Autodesk Inventor part; units mm, degrees
ref_plane "YZ Plane" through (0, 0, 0) normal (1, 0, 0) x (0, 1, 0)
ref_plane "XZ Plane" through (0, 0, 0) normal (0, 1, 0) x (-1, 0, 0)
ref_plane "XY Plane" through (0, 0, 0) normal (0, 0, 1) x (1, 0, 0)
sketch "Sketch1" plane through (0, 0, 0) normal (0, 1, 0) x (-1, 0, 0)
  line L0 (606, 0) -> (606, -30)
  arc A0 (571.724, -77.4632) -> (606, -30) centre (556, -30) ccw
  arc A1 (0, -169.7009) -> (571.724, -77.4632) centre (0, 1648.2991) ccw
  line L1 (0, 191.6842) -> (0, -191.6842)
  arc A2 (0, -163.7009) -> (569.8371, -71.7676) centre (0, 1648.2991) ccw
  arc A3 (569.8371, -71.7676) -> (600, -30) centre (556, -30) ccw
  line L2 (600, -30) -> (600, 0)
  line L3 (600, 0) -> (606, 0)
  line L4 (0, -163.7009) -> (0, -169.7009)
  point P0 (0, 0)
  point P1 (0, 0)
  point P2 (0, -166.7009)
  point P3 (0, -163.7009)
  point P4 (0, -169.7009)
  dimension "d0" = 50
  dimension "d1" = 30
  dimension "d3" = 1818
  dimension "d4" = 606
  dimension "d6" = 6
revolve "Revolution1" add sketch "Sketch1" angle 360 about axis through (0, 0, 191.6842) along (0, 0, -1)
sketch "Sketch2" plane through (0, 0, 0) normal (0, 0, 1) x (1, 0, 0)
  circle A0 centre (0, 0) radius 16.75
  dimension "d8" = 33.5
extrude "Extrusion1" cut sketch "Sketch2" against normal through all
properties part number "Сферическое дно D1000"
For this review, take the finished solid that the model builds, in its own axes (mm). Coordinates: 2 decimals unless noted, no trailing zeros. Write each loop counter-clockwise with the first axis right and the second up, starting at its lowest first coordinate (ties: lowest second). Pieces come first, ordered by that corner, then holes. Notation, with made-up numbers: (-29, 61) - (-6, 61) arc R28 cw to (-6, 97) - close; hole circle Ø9 at (23, -12.75). An arc over 180 degrees is marked (long way). Answer in a Markdown table with one row per item. Add a question column.
Q1. For P1, Ø10, axis at x = -359, y = -318, coming from the +Z side; P2, Ø3, axis at x = -34.5, y = 238, coming from the +Z side; P3, Ø6, axis at x = 460, z = -27.5, coming from the +Y side, all flat-tipped, find the tip position at first contact; note any pin that passes through.
Q2. We need section A-A, the plane z = -50. State the section outline as (x, y) points, and give its area (3 significant figures).
Q3. Draft analysis for pull direction Y (two halves, no side actions). For faces 1 (the cylindrical face through (605.414, 26.645, -15.21)), 2 (the flat face through (586, 137, 0)), 3 (the cylindrical face through (-3.63, -16.35, -166.58)), state which applies: +Y half, -Y half, draft (parallel to the pull), parting line (faces both ways), or undercut.
Q4. For probe 1 along Y at (x, z) = (0, -10.25); probe 2 along Y at (x, z) = (-109, -18); probe 3 along X at (y, z) = (-284, -20), list the stretches that pass through material, from the lowest coordinate up.
Answer list:
| question | item | result |
|---|---|---|
| 1 | P1 | stops at z = -97.7 |
| 1 | P2 | stops at z = -147.47 |
| 1 | P3 | stops at y = 397.98 |
| 2 | outline | circle Ø1203.65 at (0, 0); hole circle Ø1190.38 at (0, 0) |
| 2 | area | 24,900 mm2 |
| 3 | face 1 | parting line |
| 3 | face 2 | draft |
| 3 | face 3 | undercut |
| 4 | probe 1 | y = -606 to -600, 600 to 606 |
| 4 | probe 2 | y = -596.12 to -590.02, 590.02 to 596.12 |
| 4 | probe 3 | x = -535.33 to -528.53, 528.53 to 535.33 |
